Geometry check sheet. Reference: the model listing, model coordinates, mm. A direction names the side the tool comes from. Give positions to 0.01 mm unless a question says otherwise; leave off trailing zeros. Loops run counter-clockwise (first coordinate to the right, second up) from the corner with the lowest first, then second, coordinate; pieces in that order, holes last. Notation, with made-up numbers: (-9.75, -7) -> (34.25, -7) arc R19 ccw to (34.25, 9) -> close; hole circle Ø8 at (33, 19.25). An arc over 180 degrees is marked (long way). Answer as a JSON object with one key per item and string values.
from build123d import *

# Parameters (mm, degrees)
SKETCH1_R           = 2.25
BOSS_EXTRUDE1_DEPTH = 6
FILLET1_R           = 4


with BuildPart() as part:
    # Sketch1 → Boss-Extrude1 (new body)
    with BuildSketch(Plane(origin=(0, 0, 0), x_dir=(1, 0, 0), z_dir=(0, 1, 0))):
        Polygon((-71.479040749, 49.048444694), (-71.479040749, 9.048444694), (-41.934808158, 3.838999364), (-107.848225403, -20.151522552), (-105.112064256, -27.669063518), (-11.142802178, 6.532950815), (-63.479040749, 15.761241744), (-63.479040749, 49.048444694), align=None)
        with Locations(Location((-67.479040749, 44.077475717, 0), (0, 0, 270))):
            Circle(SKETCH1_R, mode=Mode.SUBTRACT)
        Polygon((-38.433012349, 5.25170526), (-38.433012349, 3.55170526), (-37.083012349, 3.55170526), (-37.083012349, 2.20170526), (-35.383012349, 2.20170526), (-35.383012349, 3.55170526), (-34.033012349, 3.55170526), (-34.033012349, 5.25170526), (-35.383012349, 5.25170526), (-35.383012349, 6.60170526), (-37.083012349, 6.60170526), (-37.083012349, 5.25170526), align=None, mode=Mode.SUBTRACT)
    extrude(amount=BOSS_EXTRUDE1_DEPTH)

    # Fillet1
    fillet1_edges = [part.edges().sort_by_distance(p)[0] for p in [
        (-63.479040749, 3, -15.761241744),
        (-71.479040749, 3, -9.048444694),
        (-105.112064256, 3, 27.669063518),
        (-107.848225403, 3, 20.151522552),
        (-41.934808158, 3, -3.838999364),
        (-11.142802178, 3, -6.532950815),
        (-63.479040749, 3, -49.048444694),
        (-71.479040749, 3, -49.048444694),
    ]]
    fillet(fillet1_edges, radius=FILLET1_R - 0.0001)  # a hair under: the kernel refuses the full size


solid = part.part
1) Material ranges on line 1 along X through (y, z) = (2.6, -32); line 2 along Z through (x, y) = (-66.5, 3.3); line 3 along X through (y, z) = (0.85, -44.5), recorded low to high. Write a range as from..to.
Geometry check:
{"line 1": "x = -71.48..-63.48", "line 2": "z = -48.93..-46.1, -42.05..-8.17, 5.1..13.62", "line 3": "x = -71.48..-69.69, -65.27..-63.48"}
2) Section check B-B on y = 3. Count the separate pieces of the cut face and the enclosed holes in it, plus the area to 3 significant figures.
Geometry check:
{"separate pieces": "1", "enclosed holes": "2", "area": "1,260 mm2"}
3) Draft check along X on faces 6 (the face through (-104.45, 3.04, 26.15)), 7 (the face through (-22.56, 3.04, -5.61)), 8 (the face through (-36, 3, -6.602)). Enter one of: pulls with the +X half, pulls with the -X half, needs draft (parallel to the pull), parting line crosses it, or undercut.
Geometry check:
{"face 6": "parting line crosses it", "face 7": "pulls with the +X half", "face 8": "undercut"}
4) Tool access check on faces 1 (the face through (-38.433, 3, -4)), 2 (the face through (-70.6, 3, -9.9)), 3 (the face through (-71.479, 3, -29)), 4 (the face through (-62, 6, -9)), 5 (the face through (-63.479, 3, -32)). Record the directions out of +Z, -Z, +X, -X, +Y, -Y that give a thin tool (end or side, any length) a straight path to the whole face; none if there is none.
Geometry check:
{"face 1": "+Y, -Y", "face 2": "-X, +Y, -Y", "face 3": "-Z, -X, +Y, -Y", "face 4": "+Z, -Z, +X, -X, +Y", "face 5": "-Z, +X, +Y, -Y"}
5) Section check C-C on z = -29. Record the cut outline in (x, y).
Geometry check:
{"outline": "(-71.48, 0) -> (-63.48, 0) -> (-63.48, 6) -> (-71.48, 6) -> close"}
6) Section check A-A on x = -62. Record the cut outline in (y, z), plus the area to 3 significant figures.
Geometry check:
{"outline": "(0, -16.01) -> (6, -16.01) -> (6, -7.38) -> (0, -7.38) -> close; (0, 3.46) -> (6, 3.46) -> (6, 11.98) -> (0, 11.98) -> close", "area": "103 mm2"}
7) Depth check by flat-ended pin: P1, Ø0.7, axis at x = -38, y = 3, coming from the +Z side; P2, Ø6, axis at x = -75.5, z = 13, coming from the -Y side; P3, Ø2, axis at x = -89.5, y = 4.5, coming from the -Z side; P4, Ø0.5, axis at x = -36, y = 3.5, coming from the -Z side. Enter the tip coordinate at first touch or a pass-through.
Geometry check:
{"P1": "stops at z = 3.37", "P2": "stops at y = 0", "P3": "stops at z = 13.11", "P4": "stops at z = -10.96"}
8) Section check D-D on x = -42. Record the cut outline in (y, z), plus the area to 3 significant figures.
Geometry check:
{"outline": "(0, -11.97) -> (6, -11.97) -> (6, 4.7) -> (0, 4.7) -> close", "area": "100 mm2"}
